Geometry: final body of the model. Coordinates: model frame, mm. Face numbers are marked on the shaded views. A direction names the side the tool comes from. Coordinates: 2 decimals unless noted, no trailing zeros. Order: outer loops, then holes, each group sorted by start corner. A loop starts at its lowest first (then second) coordinate and runs counter-clockwise, first axis right, second up. Notation, with made-up numbers: M 46.25,23.25 L 61.25,23.25 A31 cw 61.25,57.25 Z; hole C 6.5,-8 d9. An arc over 180 degrees is marked long. Use CSV: the item, a comma, the result in double quotes. Start each with the question number.
Q1. Section query D-D, the plane x = 3.5. Output: boundary loops of the cut face in (y, z), and give its area (3 significant figures).
Q2. Ray query, probe 1 along Y at (x, z) = (-5.75, 22.65); probe 2 along X at (y, z) = (10.5, 8); probe 3 along Z at (x, y) = (-5, 2.75). Return the intervals inside material, ascending.
Q3. Section query B-B, the plane z = 10.5. Output: boundary loops of the cut face in (x, y), and give its area (3 significant figures).
Q4. Section query C-C, the plane x = -4.25. Output: boundary loops of the cut face in (y, z).
Q5. Section query A-A, the plane y = 7.5. Output: boundary loops of the cut face in (x, z).
Q6. First-contact query: P1, Ø4.5, axis at x = 3.5, y = 6, coming from the +Z side; P2, Ø9, axis at y = 9, z = -17.5, coming from the +X side; P3, Ø5.5, axis at x = 1.5, y = 10.5, coming from the -Z side. Flat tips, straight axial feed; report the tip coordinate or a pass-through.
Q7. Mould query, pull axis Z, two halves, no side actions, for the marked faces 5, 6, 7 and 8. Classes: +Z half, -Z half, draft (parallel to the pull), parting line (faces both ways), or undercut.
Q8. Access query for the marked faces 1, 2, 3 and 4. Directions: +Z, -Z, +X, -X, +Y, -Y. A direction counts if a zero-diameter tool reaches every point of the face in a straight line with its end or side. Return the directions, or none.
Autodesk Inventor part; units mm, degrees
ref_plane "YZ Plane" through (0, 0, 0) normal (1, 0, 0) x (0, 1, 0)
ref_plane "XZ Plane" through (0, 0, 0) normal (0, 1, 0) x (-1, 0, 0)
ref_plane "XY Plane" through (0, 0, 0) normal (0, 0, 1) x (1, 0, 0)
sketch "Sketch1" plane through (0, 0, 0) normal (0, 1, 0) x (-1, 0, 0)
  line L0 (3.5, 9.65) -> (-7.5, 9.65)
  line L1 (-7.5, 9.65) -> (-7.5, -9.65)
  line L2 (-7.5, -9.65) -> (3.5, -9.65)
  line L3 (7.5, -9.65) -> (7.5, 9.65)
  line L4 (7.5, 9.65) -> (-7.5, -9.65) construction
  line L5 (-7.5, 9.65) -> (7.5, -9.65) construction
  line L6 (3.5, 9.65) -> (3.5, 15.65)
  line L7 (3.5, 15.65) -> (7.5, 15.65)
  line L8 (7.5, 15.65) -> (7.5, 9.65)
  line L9 (-7.5, 0) -> (7.5, 0) construction
  line L10 (3.5, -9.65) -> (3.5, -15.65)
  line L11 (3.5, -15.65) -> (7.5, -15.65)
  line L12 (7.5, -15.65) -> (7.5, -9.65)
  line L13 (11.5, 9.65) -> (11.5, -9.65)
  line L14 (11.5, -9.65) -> (11.5, -19.65)
  line L15 (-0.5, -19.65) -> (-0.5, -13.65)
  line L16 (-0.5, -13.65) -> (-11.5, -13.65)
  line L17 (-11.5, -13.65) -> (-11.5, 13.65)
  line L18 (-11.5, 13.65) -> (-0.5, 13.65)
  line L19 (-0.5, 13.65) -> (-0.5, 19.65)
  line L20 (11.5, 19.65) -> (11.5, 9.65)
  line L21 (11.5, 19.65) -> (11.5, 29.65)
  line L22 (11.5, 29.65) -> (-0.5, 29.65)
  line L23 (-0.5, 29.65) -> (-0.5, 19.65)
  line L24 (11.5, -19.65) -> (11.5, -29.65)
  line L25 (11.5, -29.65) -> (-0.5, -29.65)
  line L26 (-0.5, -29.65) -> (-0.5, -19.65)
  point P0 (0, 0)
  dimension "d0" = 15
  dimension "d1" = 19.3
  dimension "d2" = 4
  dimension "d3" = 6
  dimension "d4" = 4
  dimension "d5" = 10
extrude "Extrusion1" add sketch "Sketch1" along normal blind 15
sketch "Sketch2" plane through (0.5, 0, 29.65) normal (1, 0, 0) x (0, 0, -1)
  line L0 (0, 0) -> (0, 15) construction
  line L1 (0, 7.5) -> (7, 7.5) construction
  circle A0 centre (7, 7.5) radius 2.75
  line L2 (29.65, 0) -> (29.65, 27.4912) construction
  line L3 (59.3, 7.5) -> (52.3, 7.5) construction
  circle A1 centre (52.3, 7.5) radius 2.75
  dimension "d8" = 7
  dimension "d9" = 5.5
extrude "Extrusion2" cut sketch "Sketch2" against normal blind 15
fillet "Fillet1" radius 2 18 edges at (11.5, 7.5, 13.65) (11.5, 15, 0) (6, 15, 13.65) (11.5, 0, 0) (11.5, 7.5, -13.65) (6, 0, -13.65) (6, 0, 13.65) (0.5, 15, 21.65) (0.5, 0, 21.65) (0.5, 7.5, 29.65) (0.5, 0, -21.65) (0.5, 7.5, -29.65) (0.5, 15, -21.65) (-5.5, 0, -29.65) (-5.5, 15, 29.65) (-5.5, 0, 29.65) (-5.5, 15, -29.65) (6, 15, -13.65)
properties part number "actuator_mounting"
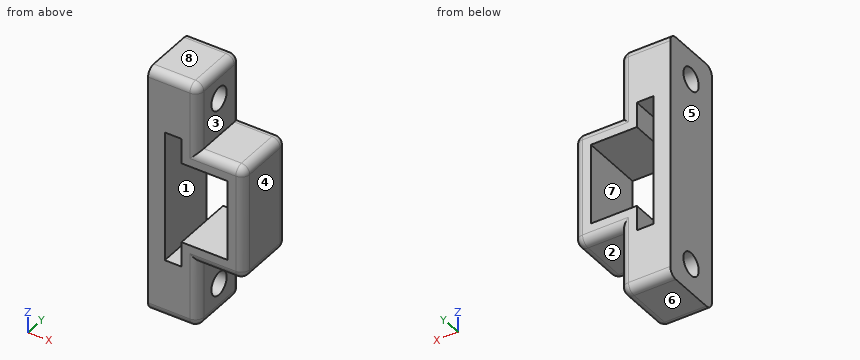
Responses:
1,outline,"M 0,-11.65 A2 ccw 2,-13.65 L 13,-13.65 A2 ccw 15,-11.65 L 15,-9.65 L 0,-9.65 Z; M 0,9.65 L 15,9.65 L 15,11.65 A2 ccw 13,13.65 L 2,13.65 A2 ccw 0,11.65 Z"
1,area,"117 mm²"
2,probe 1,"y = 0 to 4.75, 10.25 to 15"
2,probe 2,"x = -11.5 to -7.5, 7.5 to 11.5"
2,probe 3,"z = -29.65 to -15.65, 15.65 to 29.65"
3,outline,"M -11.5,0 L -7.5,0 L -7.5,15 L -11.5,15 Z; M -3.5,0 L 9.5,0 A2 ccw 11.5,2 L 11.5,13 A2 ccw 9.5,15 L -3.5,15 Z"
3,area,"283 mm²"
4,outline,"M 0,-27.65 A2 ccw 2,-29.65 L 13,-29.65 A2 ccw 15,-27.65 L 15,-15.65 L 0,-15.65 Z; M 0,15.65 L 15,15.65 L 15,27.65 A2 ccw 13,29.65 L 2,29.65 A2 ccw 0,27.65 Z; hole C 7.5,-22.65 d5.5; hole C 7.5,22.65 d5.5"
5,outline,"M -11.5,-29.65 L -1.5,-29.65 A2 ccw 0.5,-27.65 L 0.5,-25.4 L -11.5,-25.4 Z; M -11.5,-19.9 L 0.5,-19.9 L 0.5,-13.65 L 9.5,-13.65 A2 ccw 11.5,-11.65 L 11.5,11.65 A2 ccw 9.5,13.65 L 0.5,13.65 L 0.5,19.9 L -11.5,19.9 Z; M -11.5,25.4 L 0.5,25.4 L 0.5,27.65 A2 ccw -1.5,29.65 L -11.5,29.65 Z; hole M -7.5,-15.65 L -3.5,-15.65 L -3.5,-9.65 L 7.5,-9.65 L 7.5,9.65 L -3.5,9.65 L -3.5,15.65 L -7.5,15.65 Z"
6,P1,"stops at z = 13.65"
6,P2,"stops at x = 10.98"
6,P3,"stops at z = -29.63"
7,face 5,"draft"
7,face 6,"-Z half"
7,face 7,"undercut"
7,face 8,"+Z half"
8,face 1,"+Y, -Y"
8,face 2,"-Z, +X, +Y, -Y"
8,face 3,"+Z, +X, +Y, -Y"
8,face 4,"+Z, -Z, +X, +Y, -Y"
